from build123d import *

# Parameters (mm, degrees)
SKETCH1_W               = 30
SKETCH1_H               = 20
SKETCH1_R               = 1.25
BOSS_EXTRUDE1_DEPTH     = 1
SKETCH2_W               = 10
SKETCH2_H               = 12
BOSS_EXTRUDE2_DEPTH     = 2.5
SKETCH3_R               = 1.5
SKETCH3_R_2             = 1.25
SKETCH3_RX              = 0.916848001
SKETCH3_RY              = 0.710785017
SKETCH3_R_3             = 0.45
BOSS_EXTRUDE3_DEPTH     = 0.25
SKETCH4_R               = 0.45
CUT_EXTRUDE1_DEPTH      = 3.5
CUT_EXTRUDE1_DEPTH_BACK = 5


with BuildPart() as part:
    # Sketch1 → Boss-Extrude1 (new body)
    with BuildSketch(Plane(origin=(0, 0, 0), x_dir=(1, 0, 0), z_dir=(0, 1, 0))):
        Rectangle(SKETCH1_W, SKETCH1_H)
        with Locations((-12, 7)):
            Circle(SKETCH1_R, mode=Mode.SUBTRACT)
        with Locations((12, 7)):
            Circle(SKETCH1_R, mode=Mode.SUBTRACT)
        with Locations((12, -7)):
            Circle(SKETCH1_R, mode=Mode.SUBTRACT)
        with Locations((-12, -7)):
            Circle(SKETCH1_R, mode=Mode.SUBTRACT)
        with Locations((12, -2)):
            Circle(SKETCH1_R, mode=Mode.SUBTRACT)
    extrude(amount=BOSS_EXTRUDE1_DEPTH)

    # Sketch2 → Boss-Extrude2 (add)
    with BuildSketch(Plane(origin=(0, 0, 0), x_dir=(1, 0, 0), z_dir=(0, 1, 0))):
        with Locations((0, 2.22835765)):
            Rectangle(SKETCH2_W, SKETCH2_H)
    extrude(amount=BOSS_EXTRUDE2_DEPTH)

    # Sketch3 → Boss-Extrude3 (add)
    with BuildSketch(Plane(origin=(0, 1, 0), x_dir=(1, 0, 0), z_dir=(0, 1, 0))):
        with Locations((-12, 7)):
            Circle(SKETCH3_R)
        with Locations((-12, 7)):
            Circle(SKETCH3_R_2, mode=Mode.SUBTRACT)
        with Locations((12, 7)):
            Circle(SKETCH3_R)
        with Locations((12, 7)):
            Circle(SKETCH3_R_2, mode=Mode.SUBTRACT)
        with Locations((12, -7)):
            Circle(SKETCH3_R)
        with Locations((12, -7)):
            Circle(SKETCH3_R_2, mode=Mode.SUBTRACT)
        with Locations((-12, -7)):
            Circle(SKETCH3_R)
        with Locations((-12, -7)):
            Circle(SKETCH3_R_2, mode=Mode.SUBTRACT)
        with Locations((-13.5, 3.81)):
            Ellipse(SKETCH3_RX, SKETCH3_RY)
        with Locations((-13.5, 3.81)):
            Circle(SKETCH3_R_3, mode=Mode.SUBTRACT)
        with Locations((-13.5, 1.27)):
            Ellipse(SKETCH3_RX, SKETCH3_RY)
        with Locations((-13.5, 1.27)):
            Circle(SKETCH3_R_3, mode=Mode.SUBTRACT)
        with Locations((-13.5, -1.27)):
            Ellipse(SKETCH3_RX, SKETCH3_RY)
        with Locations((-13.5, -1.27)):
            Circle(SKETCH3_R_3, mode=Mode.SUBTRACT)
        with Locations((-13.5, -3.81)):
            Ellipse(SKETCH3_RX, SKETCH3_RY)
        with Locations((-13.5, -3.81)):
            Circle(SKETCH3_R_3, mode=Mode.SUBTRACT)
    extrude(amount=BOSS_EXTRUDE3_DEPTH)

    # Sketch4 → Cut-Extrude1 (cut, two sides)
    with BuildSketch(Plane(origin=(0, 0, 0), x_dir=(1, 0, 0), z_dir=(0, 1, 0))) as cut_extrude1_sk:
        with Locations((-13.5, 3.81)):
            Circle(SKETCH4_R)
        with Locations((-13.5, 1.27)):
            Circle(SKETCH4_R)
        with Locations((-13.5, -1.27)):
            Circle(SKETCH4_R)
        with Locations((-13.5, -3.81)):
            Circle(SKETCH4_R)
    extrude(amount=CUT_EXTRUDE1_DEPTH, mode=Mode.SUBTRACT)
    extrude(cut_extrude1_sk.sketch, amount=-CUT_EXTRUDE1_DEPTH_BACK, mode=Mode.SUBTRACT)


solid = part.part
Here's how the part is built. I have some questions about the finished solid (model axes, mm). A direction names the side the tool comes from. Coordinates: 2 decimals unless noted, no trailing zeros. Write each loop counter-clockwise with the first axis right and the second up, starting at its lowest first coordinate (ties: lowest second). Pieces come first, ordered by that corner, then holes.
1) If we section it at B-B (x = -12): List the corners of the cut face in (y, z) for me.
Filled in:
outline: (0, -10) - (1, -10) - (1, -8.5) - (1.25, -8.5) - (1.25, -8.25) - (0, -8.25) - close; (0, -5.75) - (1.25, -5.75) - (1.25, -5.5) - (1, -5.5) - (1, 5.5) - (1.25, 5.5) - (1.25, 5.75) - (0, 5.75) - close; (0, 8.25) - (1.25, 8.25) - (1.25, 8.5) - (1, 8.5) - (1, 10) - (0, 10) - close
2) Which directions (+Z, -Z, +X, -X, +Y, -Y) give clear straight access to the entire face, cutting with the end or side of a thin tool? Please do faces 4 (the face through (-12.99, 0.62, 7.76)), 5 (the face through (0, 2, -8.228)).
Filled in:
face 4: +Y, -Y
face 5: -Z, +Y
3) Thinking about a two-plate mould opening in X: for faces 1 (the face through (-13.29, 0.62, -0.87)), 2 (the face through (-0.2, 0.5, 10)), 3 (the face through (-15, 0.5, 0.1)), which applies, +X half, -X half, draft (parallel to the pull), parting line (faces both ways), or undercut?
Filled in:
face 1: undercut
face 2: draft
face 3: -X half
4) If we section it at D-D (x = 12): List the corners of the cut face in (y, z) for me, plus the area to 4 significant figures.
Filled in:
outline: (0, -10) - (1, -10) - (1, -8.5) - (1.25, -8.5) - (1.25, -8.25) - (0, -8.25) - close; (0, -5.75) - (1.25, -5.75) - (1.25, -5.5) - (1, -5.5) - (1, 0.75) - (0, 0.75) - close; (0, 3.25) - (1, 3.25) - (1, 5.5) - (1.25, 5.5) - (1.25, 5.75) - (0, 5.75) - close; (0, 8.25) - (1.25, 8.25) - (1.25, 8.5) - (1, 8.5) - (1, 10) - (0, 10) - close
area: 12.75 mm2
5) If we section it at A-A (y = 0.6): Count the separate pieces of the cut face and the enclosed holes in it, plus the area to 3 significant figures.
Filled in:
separate pieces: 1
enclosed holes: 9
area: 573 mm2
6) If we section it at C-C (z = -7): List the corners of the cut face in (x, y) for me.
Filled in:
outline: (-15, 0) - (-13.25, 0) - (-13.25, 1.25) - (-13.5, 1.25) - (-13.5, 1) - (-15, 1) - close; (-10.75, 0) - (10.75, 0) - (10.75, 1.25) - (10.5, 1.25) - (10.5, 1) - (5, 1) - (5, 2.5) - (-5, 2.5) - (-5, 1) - (-10.5, 1) - (-10.5, 1.25) - (-10.75, 1.25) - close; (13.25, 0) - (15, 0) - (15, 1) - (13.5, 1) - (13.5, 1.25) - (13.25, 1.25) - close
7) I'm going to push flat-ended pins straight in: pin 1 (0.8 mm diameter, centred on x = 0, y = 1.5, fed in from +Z); pin 2 (0.7 mm diameter, centred on x = -13.5, z = 1, fed in from +Y); pin 3 (3 mm diameter, centred on x = 3, z = -8, fed in from -Y); pin 4 (1.5 mm diameter, centred on y = 2, z = 0, fed in from +X). Where does each tip first touch, or does it pass through?
Filled in:
pin 1: stops at z = 3.77
pin 2: stops at y = 1.25
pin 3: stops at y = 0
pin 4: stops at x = 5
8) If I drill on line 1 (Z direction, x = -13.5, y = 0.35); line 2 (Z direction, x = 12, y = 0.75); line 3 (Z direction, x = -12, y = 0.85), over which ranges is the centre line in solid material (lowest first)?
Filled in:
line 1: z = -10 to -4.26, -3.36 to -1.72, -0.82 to 0.82, 1.72 to 3.36, 4.26 to 10
line 2: z = -10 to -8.25, -5.75 to 0.75, 3.25 to 5.75, 8.25 to 10
line 3: z = -10 to -8.25, -5.75 to 5.75, 8.25 to 10
